Study the drawing (mm; zero at the part's minimum x, y, z) and answer. A direction names the side the tool comes from. Give positions to 0.01 mm unless a question says otherwise; leave off trailing zeros. Order: outer loops, then holes, each group sorted by start corner. A loop starts at its lowest first (then second) coordinate and runs counter-clockwise, first axis right, second up. Notation, with made-up numbers: (69.25, 29.5) -> (102.25, 29.5) arc R15 ccw to (102.25, 44.5) -> close; hole circle Ø1 at (-24.75, -26.75). An arc over 180 degrees is marked (long way). One line per question, with ' | ' between items. Start each with the question number.
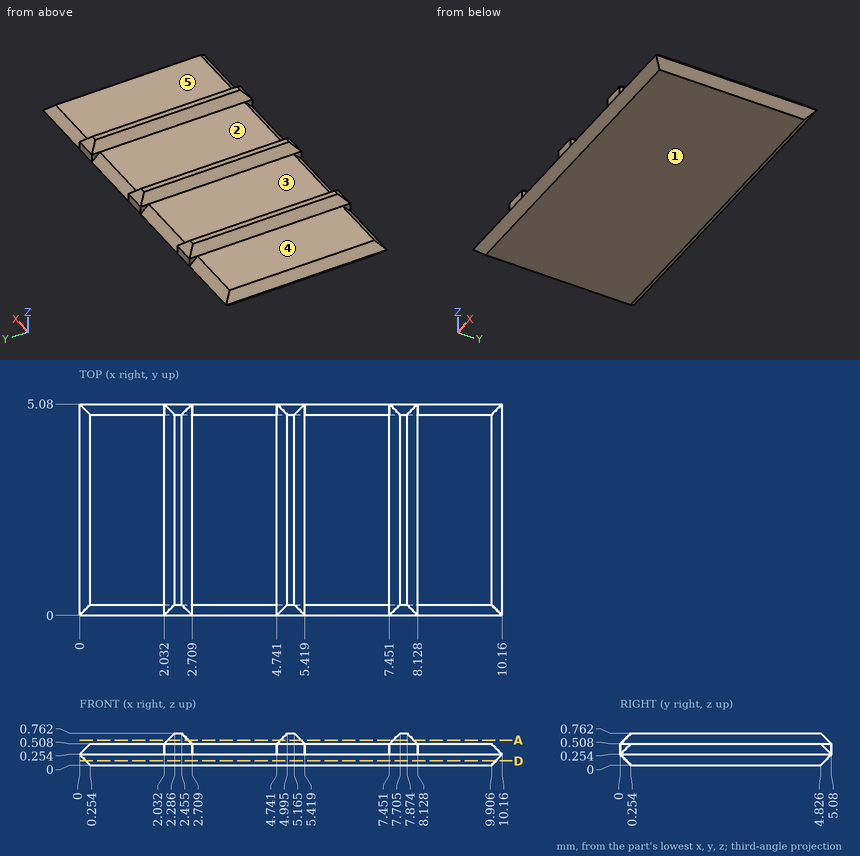
Q1. Which of the six approach directions +Z, -Z, +X, -X, +Y, -Y give full straight-line access (tool end or side, diameter ignored) to the marked faces 3, 4 and 5?
Q2. Given P1, Ø1, axis at x = 6.5, y = 3.5, coming from the +Z side; P2, Ø0.9, axis at x = 8.5, y = 3.5, coming from the +Z side (1 decimal), each flat-ended and moving along its own axis, determine where each tip first touches the part or whether it passes through.
Q3. Determine the mould class of the marked faces 1 and 2 for opening direction X: pulls with the +X half, pulls with the -X half, needs draft (parallel to the pull), parting line crosses it, or undercut.
Q4. A cutting plane is placed at A-A, the plane z = 0.6. Determine the outline of the cut face in (x, y).
Q5. A cutting plane is placed at D-D, the plane z = 0.1. Determine the outline of the cut face in (x, y), then the cut area to 3 significant figures.
Q6. Find the intervals of material crossed by line 1 (X direction, y = 3.3, z = 0.55) (1 decimal); line 2 (Z direction, x = 6.5, y = 2); line 3 (X direction, y = 1.5, z = 0.7) (1 decimal), in increasing order.
Geometry results:
1) face 3: +Z, +Y, -Y | face 4: +Z, -X, +Y, -Y | face 5: +Z, +X, +Y, -Y
2) P1: z = 0.51 | P2: z = 0.6
3) face 1: needs draft | face 2: undercut
4) outline: (2.12, 0.09) -> (2.62, 0.09) -> (2.62, 4.99) -> (2.12, 4.99) -> close; (4.83, 0.09) -> (5.33, 0.09) -> (5.33, 4.99) -> (4.83, 4.99) -> close; (7.54, 0.09) -> (8.04, 0.09) -> (8.04, 4.99) -> (7.54, 4.99) -> close
5) outline: (0.15, 0.15) -> (10.01, 0.15) -> (10.01, 4.93) -> (0.15, 4.93) -> close | area: 47.0 mm²
6) line 1: 2.1 to 2.7, 4.8 to 5.4, 7.5 to 8.1 | line 2: 0 to 0.51 | line 3: 2.2 to 2.5, 4.9 to 5.2, 7.6 to 7.9
